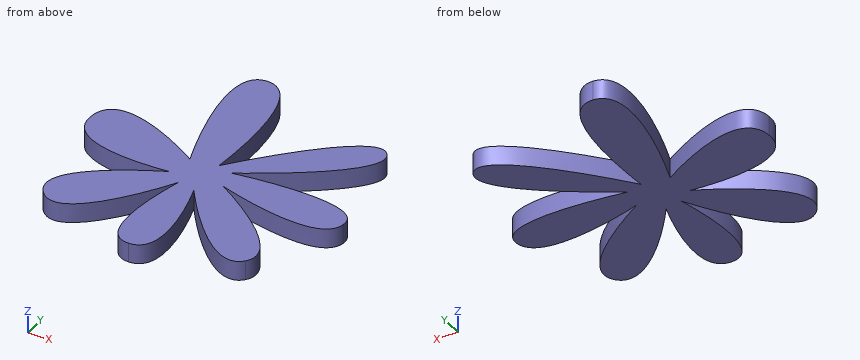
from build123d import *

# Parameters (mm, degrees)
EXTRUDE_DEPTH = 10


with BuildPart() as part:
    # path4138 → Extrude (new body)
    with BuildSketch(Plane(origin=(6.216936, 7.457358, 0), x_dir=(0, -1, 0), z_dir=(0, 0, -1))):
        with BuildLine():
            add(Edge.make_bspline(
                [(-0.397465, 15.756072), (-0.397465, 15.756072), (-72.735897, 42.783617), (-73.133362, 18.935779)],
                knots=[0, 0, 0, 0, 1, 1, 1, 1], degree=3))
            add(Edge.make_bspline(
                [(-73.133362, 18.935779), (-73.530824, -4.912055), (-2.384783, 1.844833), (-2.384783, 1.844833)],
                knots=[0, 0, 0, 0, 1, 1, 1, 1], degree=3))
            add(Edge.make_bspline(
                [(-2.384783, 1.844833), (-2.384783, 1.844833), (-64.389155, -46.248299), (-49.285525, -57.774754)],
                knots=[0, 0, 0, 0, 1, 1, 1, 1], degree=3))
            add(Edge.make_bspline(
                [(-49.285525, -57.774754), (-34.181898, -69.301206), (0, -6.104444), (0, -6.104444)],
                knots=[0, 0, 0, 0, 1, 1, 1, 1], degree=3))
            add(Edge.make_bspline(
                [(0, -6.104444), (0, -6.104444), (-10.731525, -73.673308), (10.731526, -70.891063)],
                knots=[0, 0, 0, 0, 1, 1, 1, 1], degree=3))
            add(Edge.make_bspline(
                [(10.731526, -70.891063), (32.194576, -68.108814), (11.128991, -8.48923), (11.128991, -8.48923)],
                knots=[0, 0, 0, 0, 1, 1, 1, 1], degree=3))
            add(Edge.make_bspline(
                [(11.128991, -8.48923), (11.128991, -8.48923), (42.926102, -61.749391), (58.824659, -48.633082)],
                knots=[0, 0, 0, 0, 1, 1, 1, 1], degree=3))
            add(Edge.make_bspline(
                [(58.824659, -48.633082), (74.723216, -35.516773), (20.668124, 1.049906), (20.668124, 1.049906)],
                knots=[0, 0, 0, 0, 1, 1, 1, 1], degree=3))
            add(Edge.make_bspline(
                [(20.668124, 1.049906), (20.668124, 1.049906), (73.530824, -17.233434), (73.133362, 3.832152)],
                knots=[0, 0, 0, 0, 1, 1, 1, 1], degree=3))
            add(Edge.make_bspline(
                [(73.133362, 3.832152), (72.732307, 25.088046), (18.680803, 10.191575), (18.680803, 10.191575)],
                knots=[0, 0, 0, 0, 1, 1, 1, 1], degree=3))
            add(Edge.make_bspline(
                [(18.680803, 10.191575), (18.680803, 10.191575), (76.313072, 41.193764), (56.83734, 57.887248)],
                knots=[0, 0, 0, 0, 1, 1, 1, 1], degree=3))
            add(Edge.make_bspline(
                [(56.83734, 57.887248), (37.361608, 74.580732), (13.116309, 18.140852), (13.116309, 18.140852)],
                knots=[0, 0, 0, 0, 1, 1, 1, 1], degree=3))
            add(Edge.make_bspline(
                [(13.116309, 18.140852), (13.116309, 18.140852), (19.423121, 73.673308), (-7.949277, 71.798483)],
                knots=[0, 0, 0, 0, 1, 1, 1, 1], degree=3))
            add(Edge.make_bspline(
                [(-7.949277, 71.798483), (-36.964146, 69.811165), (-0.397465, 15.756072), (-0.397465, 15.756072)],
                knots=[0, 0, 0, 0, 1, 1, 1, 1], degree=3))
        make_face()
    extrude(amount=-EXTRUDE_DEPTH)


solid = part.part
Read the model definition and answer for the solid it produces. Units are mm, in the model's axes. Coordinates: 2 decimals unless noted, no trailing zeros. Write item = value, one per line. Start each with the question number.
1) The part is cut by section A-A, the plane x = -15. State how many separate pieces and enclosed holes the cut face has, plus the area to 3 significant figures.
2) Given P1, Ø3, axis at y = 12.5, z = 8, coming from the +X side; P2, Ø4, axis at y = -20.5, z = 6, coming from the +X side; P3, Ø6, axis at y = -41.5, z = 5.5, coming from the +X side, each flat-ended and moving along its own axis, determine where each tip first touches the part or whether it passes through.
3) Find the intervals of material crossed by L1, parallel to X at y = -49, z = 5.5; L2, parallel to X at y = -43.5, z = 3.75; L3, parallel to Y at x = 50, z = 2.25, in increasing order. Write a range as from..to.
Result:
q1.separate_pieces = 3
q1.enclosed_holes = 0
q1.area = 950 mm²
q2.P1 = 23.62
q2.P2 = 40.79
q2.P3 = 56.87
q3.L1 = -51.99..-32.99, -8.93..12.52, 36.75..56.28
q3.L2 = -54.6..-26.81, -9.03..12.17, 30.29..56.72
q3.L3 = -54.21..-31.62, -12.28..10.08, 32.22..55.9
